Design review of the part built by this model. Coordinates are the model's own, in mm. Face numbers are marked on the shaded views. Round coordinates to 2 decimals unless told otherwise and drop trailing zeros. Order: outer loops, then holes, each group sorted by start corner. A loop starts at its lowest first (then second) coordinate and runs counter-clockwise, first axis right, second up. Notation, with made-up numbers: (71, 73) - (90, 73) arc R22 cw to (90, 104) - close; hole circle Ø1 at (-5, 33). An arc over 180 degrees is marked (long way). Write item = value, one per line.
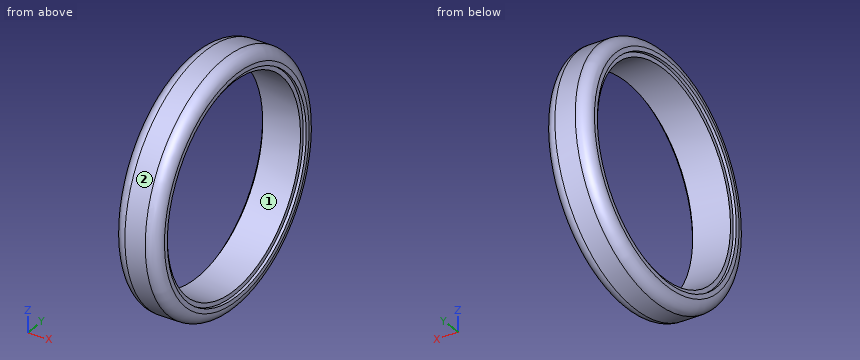
from build123d import *


with BuildPart() as part:
    # Sketch1 → Revolve1 (revolve)
    with BuildSketch(Plane.XY, mode=Mode.PRIVATE) as revolve1_sk:
        with BuildLine():
            Line((-3.5, 42), (3.5, 42))
            ThreePointArc((3.5, 42), (6.328427125, 40.828427125), (7.5, 38))
            Line((7.5, 38), (7.5, 36.5))
            Line((7.5, 36.5), (6.5, 36.5))
            Line((6.5, 36.5), (6.5, 35))
            Line((6.5, 35), (-6.5, 35))
            Line((-6.5, 35), (-6.5, 36.5))
            Line((-6.5, 36.5), (-7.5, 36.5))
            Line((-7.5, 36.5), (-7.5, 38))
            ThreePointArc((-7.5, 38), (-6.328427125, 40.828427125), (-3.5, 42))
        make_face()
        Polygon((-2.542209765, 42), (-3.292209765, 42), (-3.292209765, 41), (-1.792209765, 41), (-1.792209765, 42), align=None)
        Polygon((3.207790235, 41), (3.207790235, 42), (2.457790235, 42), (1.707790235, 42), (1.707790235, 41), align=None)
    revolve(revolve1_sk.sketch.rotate(Axis((-13.410818461, 0, 0), (1, 0, 0)), 90), axis=Axis((-13.410818461, 0, 0), (1, 0, 0)))


solid = part.part
1) The part is to be moulded in two halves that separate along Z. For the marked faces 1 and 2, say which applies: released by +Z, released by -Z, zero draft, split by the parting line, or undercut.
Findings:
face_1 = undercut
face_2 = split by the parting line
2) To check wall thickness, follow L1, parallel to Y at x = -0.5, z = 0; L2, parallel to Y at x = -4.5, z = -29.5; L3, parallel to Z at x = -5.75, y = 18. State the ranges of each line that lie inside material, in increasing order. Write a range as from..to.
Findings:
L1 = -42..-35, 35..42
L2 = -29.72..-18.83, 18.83..29.72
L3 = -37.18..-30.02, 30.02..37.18
3) We need section C-C on x = -2.25. Write out the cut boundary in (y, z).
Findings:
outline = circle Ø84 at (0, 0); hole circle Ø70 at (0, 0)
4) We need section A-A on y = 0. Write out the cut boundary in (x, z), and give its area (3 significant figures).
Findings:
outline = (-7.5, -38) arc R4 ccw to (-3.5, -42) - (3.5, -42) arc R4 ccw to (7.5, -38) - (7.5, -36.5) - (6.5, -36.5) - (6.5, -35) - (-6.5, -35) - (-6.5, -36.5) - (-7.5, -36.5) - close; (-7.5, 36.5) - (-6.5, 36.5) - (-6.5, 35) - (6.5, 35) - (6.5, 36.5) - (7.5, 36.5) - (7.5, 38) arc R4 ccw to (3.5, 42) - (-3.5, 42) arc R4 ccw to (-7.5, 38) - close
area = 190 mm^2
5) Clearance check with flat-ended pins moving along their axes: pin 1 Ø5 at (x, y) = (-1, -7.5) entering from -Z; pin 2 Ø4 at (x, z) = (3, 26.5) entering from +Y; pin 3 Ø1.5 at (x, z) = (-0.5, 15) entering from +Y. State where each tip first meets the part, or that it passes through.
Findings:
pin_1 = -41.7
pin_2 = 34.11
pin_3 = 39.51
